from build123d import *

# Parameters (mm, degrees)
SKETCH1_R           = 4.49961
BOSS_EXTRUDE2_DEPTH = 6.35
FILLET2_R           = 3.175


with BuildPart() as part:
    # Sketch1 → Boss-Extrude2 (new body)
    with BuildSketch(Plane.XY):
        with BuildLine():
            Line((77.050738686, 3.175), (5.499261314, 3.175))
            ThreePointArc((5.499261314, 3.175), (-0.387658226, 6.33815597), (-5.845205819, 2.481142666))
            Line((-5.845205819, 2.481142666), (-83.166017392, -7.012659232))
            ThreePointArc((-83.166017392, -7.012659232), (-94.540020944, -11.608054959), (-82.392147061, -13.315327295))
            Line((-82.392147061, -13.315327295), (-5.071335489, -3.821525397))
            ThreePointArc((-5.071335489, -3.821525397), (0.387658226, -6.33815597), (5.499261314, -3.175))
            Line((5.499261314, -3.175), (77.050738686, -3.175))
            ThreePointArc((77.050738686, -3.175), (88.9, 0), (77.050738686, 3.175))
        make_face()
        Circle(SKETCH1_R, mode=Mode.SUBTRACT)
        with Locations((82.55, 0)):
            Circle(SKETCH1_R, mode=Mode.SUBTRACT)
        with Locations((-88.237352881, -10.834184629)):
            Circle(SKETCH1_R, mode=Mode.SUBTRACT)
    extrude(amount=-BOSS_EXTRUDE2_DEPTH)

    # Fillet2
    fillet2_edges = [part.edges().sort_by_distance(p)[0] for p in [
        (-5.845205819, 2.481142666, -3.175),
        (5.499261314, 3.175, -3.175),
        (77.050738686, 3.175, -3.175),
        (77.050738686, -3.175, -3.175),
        (5.499261314, -3.175, -3.175),
        (-5.071335489, -3.821525397, -3.175),
        (-82.392147061, -13.315327295, -3.175),
        (-83.166017392, -7.012659232, -3.175),
    ]]
    fillet(fillet2_edges, radius=FILLET2_R)


solid = part.part
The model under review builds one solid part; all positions refer to its coordinate system, in mm. A direction names the side the tool comes from. Give positions to 0.01 mm unless a question says otherwise; leave off trailing zeros. Write each loop counter-clockwise with the first axis right and the second up, starting at its lowest first coordinate (ties: lowest second). Pieces come first, ordered by that corner, then holes.
1. Draft analysis for pull direction Y (two halves, no side actions). For faces 1 (the cylindrical face through (-0.98, -4.39, -3.13)), 2 (the flat face through (-3, -4, 0)), 3 (the flat face through (-43.987, -2.202, -3.131)), state which applies: +Y half, -Y half, draft (parallel to the pull), parting line (faces both ways), or undercut.
2. Wall thickness on L1, parallel to Y at x = 82.55, z = -1.75; L2, parallel to Y at x = 75, z = -3.75 (3 decimals); L3, parallel to Y at x = 4, z = -1: over which ranges is each line inside the solid? List them lowest first.
3. Tool access review of faces 4 (the flat face through (41, -3.175, -3)), 5 (the flat face through (-3, -4, -6.35)), 6 (the flat face through (42, 3.175, -3)): name each direction out of +Z, -Z, +X, -X, +Y, -Y from which nothing blocks a thin tool from reaching the whole face with its end or side.
4. Add section A-A, the plane x = 0. Write out the cut boundary in (y, z), plus the area to 3 significant figures.
5. Add section B-B, the plane y = 0. Write out the cut boundary in (x, z).
6. Add section C-C, the plane z = -3. Write out the cut boundary in (x, y) (3 decimals), plus the area to 3 significant figures.
7. Add section D-D, the plane x = 26.5. Write out the cut boundary in (y, z) (3 decimals).
8. For P1, Ø1, axis at x = -38, z = -4, coming from the +Y side; P2, Ø2, axis at x = 37, z = -5, coming from the +Y side (3 decimals), all flat-tipped, find the tip position at first contact; note any pin that passes through.
Worked answers:
1. face 1: undercut
1. face 2: draft
1. face 3: +Y half
2. L1: y = -6.35 to -4.5, 4.5 to 6.35
2. L2: y = -3.175 to 3.175
2. L3: y = -4.93 to -2.06, 2.06 to 4.93
3. face 4: +Z, -Z, -Y
3. face 5: -Z, +X, -X, +Y, -Y
3. face 6: +Z, -Z, +Y
4. outline: (-6.35, -6.35) - (-4.5, -6.35) - (-4.5, 0) - (-6.35, 0) - close; (4.5, -6.35) - (6.35, -6.35) - (6.35, 0) - (4.5, 0) - close
4. area: 23.5 mm2
5. outline: (-26.05, -6.35) - (-4.5, -6.35) - (-4.5, 0) - (-26.05, 0) - close; (4.5, -6.35) - (78.05, -6.35) - (78.05, 0) - (4.5, 0) - close; (87.05, -6.35) - (88.9, -6.35) - (88.9, 0) - (87.05, 0) - close
6. outline: (-84.056, -6.056) arc R6.35 ccw (long way) to (-83.024, -14.459) arc R3.175 cw to (-80.804, -13.12) - (-6.66, -4.017) arc R3.175 cw to (-4.182, -4.779) arc R6.35 ccw to (4.733, -4.233) arc R3.175 cw to (7.1, -3.175) - (75.45, -3.175) arc R3.175 cw to (77.817, -4.233) arc R6.35 ccw (long way) to (77.817, 4.233) arc R3.175 cw to (75.45, 3.175) - (7.1, 3.175) arc R3.175 cw to (4.733, 4.233) arc R6.35 ccw to (-5.214, 3.625) arc R3.175 cw to (-7.434, 2.286) - (-81.578, -6.818) arc R3.175 cw to start; hole circle Ø8.999 at (-88.237, -10.834); hole circle Ø8.999 at (0, 0); hole circle Ø8.999 at (82.55, 0)
6. area: 1,130 mm2
7. outline: (-3.175, -6.35) - (3.175, -6.35) - (3.175, 0) - (-3.175, 0) - close
8. P1: stops at y = -1.41
8. P2: stops at y = 3.175
